```python
from build123d import *

# Parameters (mm, degrees)
SKETCH1_W           = 70
SKETCH1_H           = 60
BOSS_EXTRUDE1_DEPTH = 4
SKETCH2_W           = 4
SKETCH2_H           = 60
BOSS_EXTRUDE2_DEPTH = 50
SKETCH3_R           = 13
CUT_EXTRUDE1_DEPTH  = 50
SKETCH4_R           = 2
CUT_EXTRUDE2_DEPTH  = 50


with BuildPart() as part:
    # Sketch1 → Boss-Extrude1 (new body)
    with BuildSketch(Plane.XY):
        Rectangle(SKETCH1_W, SKETCH1_H)
    extrude(amount=BOSS_EXTRUDE1_DEPTH)

    # Sketch2 → Boss-Extrude2 (add)
    with BuildSketch(Plane.XY.offset(4)):
        with Locations((-33, 0)):
            Rectangle(SKETCH2_W, SKETCH2_H)
    extrude(amount=BOSS_EXTRUDE2_DEPTH)

    # Sketch3 → Cut-Extrude1 (cut)
    with BuildSketch(Plane(origin=(-31, 0, 0), x_dir=(0, 0, -1), z_dir=(1, 0, 0))):
        with Locations((-29, 0)):
            Circle(SKETCH3_R)
    extrude(amount=-CUT_EXTRUDE1_DEPTH, mode=Mode.SUBTRACT)

    # Sketch4 → Cut-Extrude2 (cut)
    with BuildSketch(Plane.XY.offset(4)):
        with Locations((-1, 20)):
            Circle(SKETCH4_R)
        with Locations((-1, -20)):
            Circle(SKETCH4_R)
    extrude(amount=-CUT_EXTRUDE2_DEPTH, mode=Mode.SUBTRACT)


solid = part.part
```
Here's how the part is built. I have some questions about the finished solid (model axes, mm). A direction names the side the tool comes from. Round coordinates to 2 decimals unless told otherwise and drop trailing zeros. Order: outer loops, then holes, each group sorted by start corner. A loop starts at its lowest first (then second) coordinate and runs counter-clockwise, first axis right, second up. Notation, with made-up numbers: M -14.75,65.25 L -6.75,65.25 A29 ccw -6.75,101.25 Z; hole C 28.25,43.25 d1. An arc over 180 degrees is marked long. Answer in a Markdown table with one row per item.
Item 1: Imagine slicing it at B-B, the plane y = 0. Write out the boundary of the cut face in (x, z), and give its area (3 significant figures).
A:
| item | result |
|---|---|
| outline | M -35,0 L 35,0 L 35,4 L -31,4 L -31,16 L -35,16 Z; M -35,42 L -31,42 L -31,54 L -35,54 Z |
| area | 376 mm2 |
Item 2: If I drill on L1, parallel to Y at x = -1, z = 3; L2, parallel to Y at x = -34.15, z = 29; L3, parallel to Z at x = -27.5, y = -6, over which ranges is the centre line in solid material (lowest first)? Write a range as from..to.
A:
| item | result |
|---|---|
| L1 | y = -30..-22, -18..18, 22..30 |
| L2 | y = -30..-13, 13..30 |
| L3 | z = 0..4 |
Item 3: Thinking about a two-plate mould opening in Y: for faces 3 (the face through (-16, -30, 3)), 4 (the face through (0, 0, 0)), 5 (the face through (-1, -18, 2)), 6 (the face through (-1, 22, 2)), which applies, +Y half, -Y half, draft (parallel to the pull), parting line (faces both ways), or undercut?
A:
| item | result |
|---|---|
| face 3 | -Y half |
| face 4 | draft |
| face 5 | undercut |
| face 6 | undercut |
Item 4: Imagine slicing it at A-A, the plane x = -1. Write out the boundary of the cut face in (y, z).
A:
| item | result |
|---|---|
| outline | M -30,0 L -22,0 L -22,4 L -30,4 Z; M -18,0 L 18,0 L 18,4 L -18,4 Z; M 22,0 L 30,0 L 30,4 L 22,4 Z |
Item 5: Imagine slicing it at D-D, the plane y = -20. Write out the boundary of the cut face in (x, z).
A:
| item | result |
|---|---|
| outline | M -35,0 L -3,0 L -3,4 L -31,4 L -31,54 L -35,54 Z; M 1,0 L 35,0 L 35,4 L 1,4 Z |
Item 6: Imagine slicing it at C-C, the plane z = 29. Write out the boundary of the cut face in (x, y), and give its area (3 significant figures).
A:
| item | result |
|---|---|
| outline | M -35,-30 L -31,-30 L -31,-13 L -35,-13 Z; M -35,13 L -31,13 L -31,30 L -35,30 Z |
| area | 136 mm2 |
Item 7: For faces 1 (the face through (35, 0, 2)), 2 (the face through (2, 0, 4)), which set-ups out of +Z, -Z, +X, -X, +Y, -Y let a thin tool reach every point of the face, with its end or its side?
A:
| item | result |
|---|---|
| face 1 | +Z, -Z, +X, +Y, -Y |
| face 2 | +Z, +X, +Y, -Y |
Item 8: I'm going to push flat-ended pins straight in: pin 1 (1.5 mm diameter, centred on y = 15, z = 16.5, fed in from +X); pin 2 (5 mm diameter, centred on x = -14.5, y = 7.5, fed in from +Z). Where does each tip first touch, or does it pass through?
A:
| item | result |
|---|---|
| pin 1 | stops at x = -31 |
| pin 2 | stops at z = 4 |
